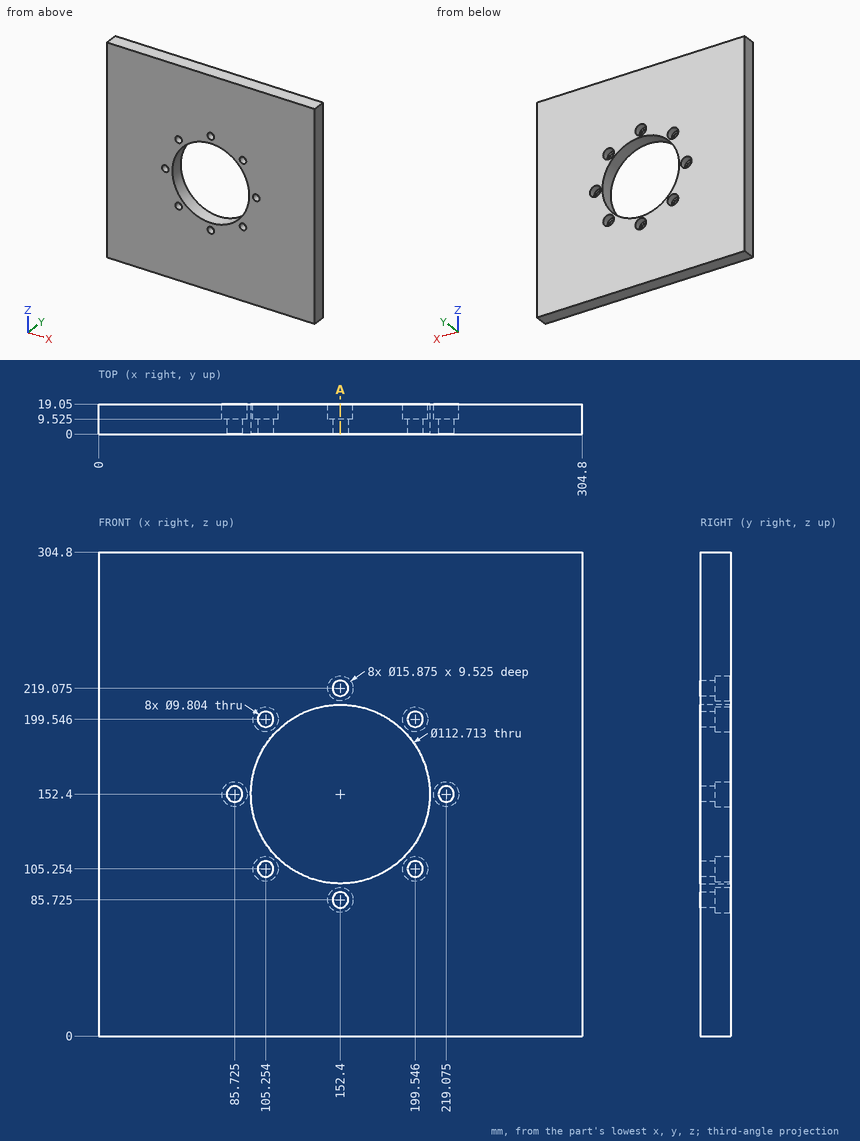
Here's the drawing with two shaded views (mm, measured from the low corner). I have some questions. Round coordinates to 2 decimals unless told otherwise and drop trailing zeros.
(1) If I drill on probe 1 along Z at (x, y) = (198, 7.25) (1 decimal); probe 2 along X at (y, z) = (14.5, 152.4); probe 3 along Z at (x, y) = (102.5, 2) (1 decimal), over which ranges is the centre line in solid material (lowest first)?
Findings below:
probe 1: z = 0 to 100.6, 109.9 to 119.3, 185.5 to 194.9, 204.2 to 304.8
probe 2: x = 0 to 77.79, 93.66 to 96.04, 208.76 to 211.14, 227.01 to 304.8
probe 3: z = 0 to 101.2, 109.3 to 126.2, 178.6 to 195.5, 203.6 to 304.8
(2) For pin 1 (11.5 mm diameter, centred on x = 152.4, z = 219.075, fed in from +Y) (1 decimal); pin 2 (6 mm diameter, centred on x = 199.55, z = 199.55, fed in from -Y), each with a flat end and sliding along its axis, tell me the tip position at first contact or that it passes through.
Findings below:
pin 1: stops at y = 9.5
pin 2: passes through
(3) Suppose I cut it at A-A on x = 152.4. State how many separate pieces and enclosed holes the cut face has, and give its area (3 significant figures).
Findings below:
separate pieces: 4
enclosed holes: 0
area: 3,170 mm2
